CAD build for the part. Positions are in the model's coordinates, mm. A direction names the side the tool comes from. Give positions to 0.01 mm unless a question says otherwise; leave off trailing zeros. Write each loop counter-clockwise with the first axis right and the second up, starting at its lowest first coordinate (ties: lowest second). Pieces come first, ordered by that corner, then holes. Notation, with made-up numbers: M 18,52.5 L 24,52.5 A29 cw 24,89.5 Z; hole C -32,55.25 d10. An arc over 180 degrees is marked long. One line per question, with ' | ' between items. Start each with the question number.
1. Cut at A-A, the plane x = -2.5. Write the cut outline in (y, z), then the cut area to 3 significant figures.
2. Cut at D-D, the plane x = 30.5. Write the cut outline in (y, z).
3. Cut at B-B, the plane z = 3.25. Write the cut outline in (x, y) (3 decimals).
4. Pull direction X, two halves, no side cores. Call faces 1 (the face through (2, 12, 0)), 2 (the face through (2, 12.802, 4)): released by +X, released by -X, zero draft, split by the parting line, or undercut.
5. Which spindle directions (+Z, -Z, +X, -X, +Y, -Y) get a long thin tool onto all of the face, cutting with end or side? Do faces 3 (the face through (2, -11.198, 4)), 4 (the face through (2, 11.262, 4)), 5 (the face through (2, 12, 8.89)). Say none if no direction does.
6. Cut at C-C, the plane y = 2.75. Write the cut outline in (x, z), then the cut area to 3 significant figures.
7. Wall check: L1, parallel to Y at x = -4, z = 5.75; L2, parallel to Y at x = -15, z = 4.25; L3, parallel to X at y = 7.5, z = 7. Give the ranges that are in metal, low to high.
8. Flat gauge pins, fed straight in: pin 1 (1 mm diameter, centred on x = 1.5, z = 2.5, fed in from +Y); pin 2 (5 mm diameter, centred on y = 12, z = 3, fed in from -X); pin 3 (2.5 mm diameter, centred on x = -2.5, z = 3.5, fed in from -Y). Where does each tip first touch, or does it go through?
```python
from build123d import *

# Parameters (mm, degrees)
F1_DEPTH = 8.89


with BuildPart() as f1:
    # F0 (on Top) → F1 (new body)
    with BuildSketch(Plane.XY):
        with BuildLine():
            Line((-18.9896195369, -11.198009608), (-19.4227703597, -11.198009608))
            Line((-19.4227703597, -11.198009608), (-19.4227703597, -7.7054101467))
            ThreePointArc((-19.4227703597, -7.7054101467), (-40.3979995929, 0.5824766479), (-19.4227703597, 8.8703634425))
            Line((-19.4227703597, 8.8703634425), (-19.4227703597, 12.6917476503))
            ThreePointArc((-19.4227703597, 12.6917476503), (-23.6180195335, 14.8405326983), (-28.2729995929, 15.5811766479))
            ThreePointArc((-28.2729995929, 15.5811766479), (-38.8786820719, 11.1881591269), (-43.2716995929, 0.5824766479))
            ThreePointArc((-43.2716995929, 0.5824766479), (-38.8786820719, -10.0232058311), (-28.2729995929, -14.4162233521))
            ThreePointArc((-28.2729995929, -14.4162233521), (-23.3603107933, -13.5888496996), (-18.9896195369, -11.198009608))
        make_face()
        with BuildLine():
            Line((-18.2107055563, -9.7378878497), (-17.3894763432, -9.7378878497))
            ThreePointArc((-17.3894763432, -9.7378878497), (-14.3410273374, -4.9728046917), (-13.2742995929, 0.5824766479))
            ThreePointArc((-13.2742995929, 0.5824766479), (-14.4361743904, 6.3706775779), (-17.7417894428, 11.2621121503))
            Line((-17.7417894428, 11.2621121503), (-18.2107055563, 11.2621121503))
            Line((-18.2107055563, 11.2621121503), (-18.2107055563, 7.3475238555))
            ThreePointArc((-18.2107055563, 7.3475238555), (-16.675134699, 4.1187394921), (-16.1479995929, 0.5824766479))
            ThreePointArc((-16.1479995929, 0.5824766479), (-16.675134699, -2.9537861963), (-18.2107055563, -6.1825705597))
            Line((-18.2107055563, -6.1825705597), (-18.2107055563, -9.7378878497))
        make_face()
        with BuildLine():
            Line((-19.4227703597, -7.7054101467), (-19.4227703597, -11.198009608))
            Line((-19.4227703597, -11.198009608), (-18.9896195369, -11.198009608))
            ThreePointArc((-18.9896195369, -11.198009608), (-18.1631535939, -10.4968742161), (-17.3894763432, -9.7378878497))
            Line((-17.3894763432, -9.7378878497), (-18.2107055563, -9.7378878497))
            Line((-18.2107055563, -9.7378878497), (-18.2107055563, -6.1825705597))
            ThreePointArc((-18.2107055563, -6.1825705597), (-18.7861326596, -6.9683498493), (-19.4227703597, -7.7054101467))
        make_face()
        with BuildLine():
            ThreePointArc((-17.3894763432, -9.7378878497), (-18.1631535939, -10.4968742161), (-18.9896195369, -11.198009608))
            Line((-18.9896195369, -11.198009608), (22.9410203511, -11.198009608))
            ThreePointArc((22.9410203511, -11.198009608), (22.1145544081, -10.4968742161), (21.3408771574, -9.7378878497))
            Line((21.3408771574, -9.7378878497), (-17.3894763432, -9.7378878497))
        make_face()
        with BuildLine():
            Line((-19.4227703597, 12.6917476503), (-19.4227703597, 8.8703634425))
            ThreePointArc((-19.4227703597, 8.8703634425), (-18.7861326596, 8.133303145), (-18.2107055563, 7.3475238555))
            Line((-18.2107055563, 7.3475238555), (-18.2107055563, 11.2621121503))
            Line((-18.2107055563, 11.2621121503), (-17.7417894428, 11.2621121503))
            ThreePointArc((-17.7417894428, 11.2621121503), (-18.5559520702, 12.0078864494), (-19.4227703597, 12.6917476503))
        make_face()
        with BuildLine():
            Line((-19.4227703597, 12.801990392), (-19.4227703597, 12.6917476503))
            ThreePointArc((-19.4227703597, 12.6917476503), (-18.5559520702, 12.0078864494), (-17.7417894428, 11.2621121503))
            Line((-17.7417894428, 11.2621121503), (21.693190257, 11.2621121503))
            ThreePointArc((21.693190257, 11.2621121503), (22.5793232744, 12.0687070475), (23.5270165736, 12.801990392))
            Line((23.5270165736, 12.801990392), (-19.4227703597, 12.801990392))
        make_face()
        with BuildLine():
            ThreePointArc((23.5270165736, 12.801990392), (22.5793232744, 12.0687070475), (21.693190257, 11.2621121503))
            Line((21.693190257, 11.2621121503), (22.2892944437, 11.2621121503))
            Line((22.2892944437, 11.2621121503), (22.2892944437, 7.5329654434))
            ThreePointArc((22.2892944437, 7.5329654434), (22.9010353132, 8.334282136), (23.5772296403, 9.0820097368))
            Line((23.5772296403, 9.0820097368), (23.5772296403, 12.801990392))
            Line((23.5772296403, 12.801990392), (23.5270165736, 12.801990392))
        make_face()
        with BuildLine():
            Line((23.5772296403, -11.198009608), (22.9410203511, -11.198009608))
            ThreePointArc((22.9410203511, -11.198009608), (27.3117115612, -13.5888496836), (32.2244003091, -14.4162233521))
            ThreePointArc((32.2244003091, -14.4162233521), (42.8300828514, -10.0232058658), (47.2231004071, 0.5824766479))
            ThreePointArc((47.2231004071, 0.5824766479), (42.8300828861, 11.1881591269), (32.2244004071, 15.5811766479))
            ThreePointArc((32.2244004071, 15.5811766479), (27.6590865682, 14.8694956246), (23.5270165736, 12.801990392))
            Line((23.5270165736, 12.801990392), (23.5772296403, 12.801990392))
            Line((23.5772296403, 12.801990392), (23.5772296403, 9.0820097368))
            ThreePointArc((23.5772296403, 9.0820097368), (36.8161690997, 11.8043875936), (44.3494004071, 0.5824766479))
            ThreePointArc((44.3494004071, 0.5824766479), (36.8161690997, -10.6394342978), (23.5772296403, -7.9170564411))
            Line((23.5772296403, -7.9170564411), (23.5772296403, -11.198009608))
        make_face()
        with BuildLine():
            ThreePointArc((21.3408771574, -9.7378878497), (22.1145544081, -10.4968742161), (22.9410203511, -11.198009608))
            Line((22.9410203511, -11.198009608), (23.5772296403, -11.198009608))
            Line((23.5772296403, -11.198009608), (23.5772296403, -7.9170564411))
            ThreePointArc((23.5772296403, -7.9170564411), (22.9010353132, -7.1693288402), (22.2892944437, -6.3680121476))
            Line((22.2892944437, -6.3680121476), (22.2892944437, -9.7378878497))
            Line((22.2892944437, -9.7378878497), (21.3408771574, -9.7378878497))
        make_face()
        with BuildLine():
            ThreePointArc((21.693190257, 11.2621121503), (17.2278107399, 0.8340716473), (21.3408771574, -9.7378878497))
            Line((21.3408771574, -9.7378878497), (22.2892944437, -9.7378878497))
            Line((22.2892944437, -9.7378878497), (22.2892944437, -6.3680121476))
            ThreePointArc((22.2892944437, -6.3680121476), (20.0994004071, 0.5824766479), (22.2892944437, 7.5329654434))
            Line((22.2892944437, 7.5329654434), (22.2892944437, 11.2621121503))
            Line((22.2892944437, 11.2621121503), (21.693190257, 11.2621121503))
        make_face()
    extrude(amount=F1_DEPTH)


solid = f1.part
```
Here are the results:
1) outline: M -11.2,0 L -9.74,0 L -9.74,8.89 L -11.2,8.89 Z; M 11.26,0 L 12.8,0 L 12.8,8.89 L 11.26,8.89 Z | area: 26.7 mm^2
2) outline: M -14.32,0 L -11.42,0 L -11.42,8.89 L -14.32,8.89 Z; M 12.58,0 L 15.48,0 L 15.48,8.89 L 12.58,8.89 Z
3) outline: M -19.423,12.692 A14.999 ccw long -18.99,-11.198 L 22.941,-11.198 A14.999 ccw long 23.527,12.802 L -19.423,12.802 Z; hole C -28.273,0.582 d24.25; hole M -17.742,11.262 A14.999 cw -17.389,-9.738 L 21.341,-9.738 A14.999 cw 21.693,11.262 Z; hole C 32.224,0.582 d24.25
4) face 1: zero draft | face 2: undercut
5) face 3: +Z, -Z, -Y | face 4: +Z, -Z | face 5: +Z, +X, -X, +Y, -Y
6) outline: M -43.11,0 L -40.2,0 L -40.2,8.89 L -43.11,8.89 Z; M -16.34,0 L -13.43,0 L -13.43,8.89 L -16.34,8.89 Z; M 17.38,0 L 20.29,0 L 20.29,8.89 L 17.38,8.89 Z; M 44.15,0 L 47.07,0 L 47.07,8.89 L 44.15,8.89 Z | area: 104 mm^2
7) L1: -11.2 to -9.74, 11.26 to 12.8 | L2: -11.2 to -9.74, -6.4 to 7.57, 11.26 to 12.8 | L3: -41.58 to -38.23, -18.31 to -14.96, 18.92 to 22.27, 42.18 to 45.53
8) pin 1: y = 12.8 | pin 2: x = -40.33 | pin 3: y = -11.2
